Build history of the part. All positions in model axes, mm. Face numbers are marked on the shaded views. A direction names the side the tool comes from. Round coordinates to 2 decimals unless told otherwise and drop trailing zeros. Loops run counter-clockwise (first coordinate to the right, second up) from the corner with the lowest first, then second, coordinate; pieces in that order, holes last. Notation, with made-up numbers: M -2,69.5 L 52,69.5 A36 cw 52,108.5 Z; hole C 4.5,79 d10. An arc over 180 degrees is marked long. Write each question's results on one line, items separated by ' | '. Start each with the question number.
```python
from build123d import *

# Parameters (mm, degrees)
SKETCH1_W           = 200
SKETCH1_H           = 75
BOSS_EXTRUDE1_DEPTH = 25
SKETCH9_W           = 165
SKETCH9_H           = 65
CUT_EXTRUDE5_DEPTH  = 4
SHELL3_START        = -34.5
SHELL3_DEPTH        = 69
SKETCH14_W          = 10
SKETCH14_H          = 10
BOSS_EXTRUDE5_DEPTH = 10
SKETCH15_R          = 5
CUT_EXTRUDE7_DEPTH  = 157.036053526
SKETCH16_W          = 20
SKETCH16_H          = 20
CUT_EXTRUDE8_DEPTH  = 157.624551077
SKETCH19_RX         = 5.75
SKETCH19_RY         = 5.5
SKETCH21_R          = 2.75
CUT_EXTRUDE9_DEPTH  = 157.624551117


# Read off the part's stored shape, not the designer's step: Shell3
with BuildPart() as part:
    # Sketch1 → Boss-Extrude1 (new body)
    with BuildSketch(Plane(origin=(0, 0, 0), x_dir=(1, 0, 0), z_dir=(0, 1, 0))):
        with Locations((40, 0)):
            Rectangle(SKETCH1_W, SKETCH1_H)
    extrude(amount=BOSS_EXTRUDE1_DEPTH)

    # Sketch9 → Cut-Extrude5 (cut)
    with BuildSketch(Plane(origin=(0, 25, 0), x_dir=(1, 0, 0), z_dir=(0, 1, 0))):
        with Locations((52.5, 0)):
            Rectangle(SKETCH9_W, SKETCH9_H)
    extrude(amount=-CUT_EXTRUDE5_DEPTH, mode=Mode.SUBTRACT)

    # Shell3 outline → Shell3 (cut)
    with BuildSketch(Plane.XY.offset(SHELL3_START)):
        Polygon((137, 0), (137, 18), (-33, 18), (-33, 22), (-60, 22), (-60, 0), align=None)
    extrude(amount=SHELL3_DEPTH, mode=Mode.SUBTRACT)

    # Sketch14 → Boss-Extrude5 (add)
    with BuildSketch(Plane(origin=(140, 0, 0), x_dir=(0, 0, -1), z_dir=(1, 0, 0))):
        with Locations((-23.5, 20)):
            Rectangle(SKETCH14_W, SKETCH14_H)
        with Locations((22.5, 20)):
            Rectangle(SKETCH14_W, SKETCH14_H)
    extrude(amount=BOSS_EXTRUDE5_DEPTH)

    # Sketch15 → Cut-Extrude7 (cut, through all)
    with BuildSketch(Plane(origin=(0, 21, 0), x_dir=(1, 0, 0), z_dir=(0, 1, 0))):
        with Locations(Location((-17.28231035, 0, 0), (0, 0, 270))):
            Circle(SKETCH15_R)
    extrude(amount=-CUT_EXTRUDE7_DEPTH, mode=Mode.SUBTRACT)

    # Sketch16 → Cut-Extrude8 (cut, through all)
    with BuildSketch(Plane(origin=(0, 25, 0), x_dir=(1, 0, 0), z_dir=(0, 1, 0))):
        with Locations((-45, 0)):
            Rectangle(SKETCH16_W, SKETCH16_H)
    extrude(amount=-CUT_EXTRUDE8_DEPTH, mode=Mode.SUBTRACT)

    # Cut-Sweep2: sweep along a path in Sketch20
    with BuildLine() as cut_sweep2_path:  # in the path sketch's own coordinates; laid on its plane below (add() does not lay a ready-made edge on the line's plane)
        add(Edge.make_bspline(
            [(-140, 6), (-136.19888528, 6.630281352), (-133.075750061, 4.182881523)],
            knots=[0, 0, 0, 1, 1, 1], degree=2))
    # Sketch19 → Cut-Sweep2 (sweep, cut)
    with BuildSketch(Plane(origin=(140, 0, 0), x_dir=(0, 0, -1), z_dir=(1, 0, 0))):
        with Locations(Location((-12.5, 6), (0, 0, 0))):
            Ellipse(SKETCH19_RX, SKETCH19_RY)
    sweep(path=Plane(origin=(0, 0, 0), x_dir=(-1, 0, 0), z_dir=(0, 0, -1)) * cut_sweep2_path.line, mode=Mode.SUBTRACT)

    # Sketch21 → Cut-Extrude9 (cut, through all)
    with BuildSketch(Plane(origin=(0, 25, 0), x_dir=(1, 0, 0), z_dir=(0, 1, 0))):
        with Locations(Location((-45, 13.5, 0), (0, 0, 270))):
            Circle(SKETCH21_R)
    extrude(amount=-CUT_EXTRUDE9_DEPTH, mode=Mode.SUBTRACT)


solid = part.part
```
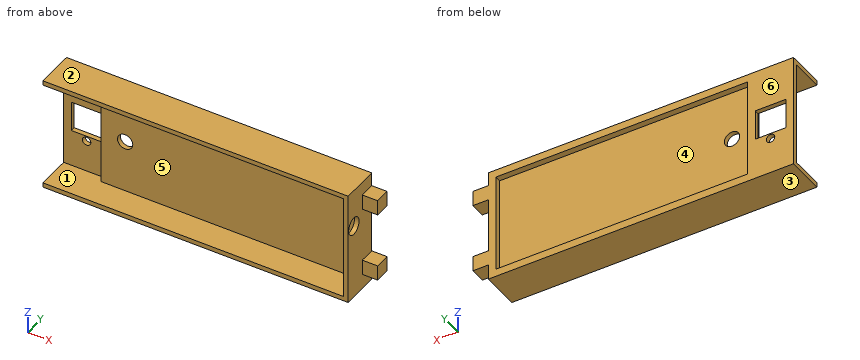
Item 1: Mould opens along Z. For the marked faces 1, 2 and 3 say: released by +Z, released by -Z, zero draft, split by the parting line, or undercut.
Item 2: Tool access for the marked faces 4, 5 and 6: list every direction of +Z, -Z, +X, -X, +Y, -Y with a clear straight run to the whole face (end or side of a thin tool).
Item 3: Saw through at A-A, the plane z = 0. Give the cut face in (x, y), then the cut area to 3 significant figures.
Item 4: Saw through at B-B, the plane x = -45. Give the cut face in (y, z).
Item 5: Saw through at C-C, the plane z = -13.5. Give the cut face in (x, y), then the cut area to 4 significant figures.
Item 6: Drop flat-ended pins along their axis: pin 1 (2 mm diameter, centred on y = 8.5, z = -6, fed in from -X); pin 2 (5 mm diameter, centred on y = 22.5, z = -28.5, fed in from +X); pin 3 (21.5 mm diameter, centred on x = -41.5, z = -14, fed in from -Y); pin 4 (5 mm diameter, centred on x = 144, y = 22, fed in from -Z). Give the stop position or say it passes through.
Item 7: Drill centre lines: line 1 along X through (y, z) = (24.35, -13.5); line 2 along X through (y, z) = (20.4, 0); line 3 along Z through (x, y) = (-18.5, 4.25). Where is each one in solid material? Low to high. Write a range as [from, to].
Item 8: Saw through at D-D, the plane x = 25. Give the cut face in (y, z).
Working result:
1) face 1: undercut | face 2: released by +Z | face 3: released by -Z
2) face 4: +Y | face 5: -X, -Y | face 6: +Z, -Z, +X, -X, +Y
3) outline: M -60,22 L -55,22 L -55,25 L -60,25 Z; M -35,22 L -33,22 L -33,18 L -22.28,18 L -22.28,21 L -30,21 L -30,25 L -35,25 Z; M -12.28,18 L 137,18 L 137,0 L 140,0 L 140,25 L 135,25 L 135,21 L -12.28,21 Z | area: 596 mm²
4) outline: M 0,-37.5 L 25,-37.5 L 25,-16.25 L 22,-16.25 L 22,-34.5 L 0,-34.5 Z; M 0,34.5 L 22,34.5 L 22,10 L 25,10 L 25,37.5 L 0,37.5 Z; M 22,-10.75 L 25,-10.75 L 25,-10 L 22,-10 Z
5) outline: M -60,22 L -47.75,22 L -47.75,25 L -60,25 Z; M -42.25,22 L -33,22 L -33,18 L 137,18 L 137,0 L 140,0 L 140,25 L 135,25 L 135,21 L -30,21 L -30,25 L -42.25,25 Z | area: 669.5 mm²
6) pin 1: stops at x = 137 | pin 2: stops at x = 150 | pin 3: stops at y = 18 | pin 4: stops at z = -27.5
7) line 1: x = [-60, -47.75], [-42.25, -30], [135, 140] | line 2: x = [-33, -22.28], [-12.28, 140] | line 3: z = [-37.5, -34.5], [34.5, 37.5]
8) outline: M 0,-37.5 L 25,-37.5 L 25,-32.5 L 21,-32.5 L 21,32.5 L 25,32.5 L 25,37.5 L 0,37.5 L 0,34.5 L 18,34.5 L 18,-34.5 L 0,-34.5 Z
